Input: part model. Units: mm. Frame: model coordinates. A direction names the side the tool comes from. Give positions to 0.01 mm unless a question says otherwise; leave off trailing zeros. Order: outer loops, then holes, each group sorted by start corner. A loop starts at its lowest first (then second) coordinate and runs counter-clockwise, first axis right, second up. Notation, with made-up numbers: M 25,26 L 48,26 A16 ccw 48,43 Z; hole C 77,70 d7. An arc over 180 degrees is marked long. Use a Markdown table: item, result.
from build123d import *

# Parameters (mm, degrees)
SKETCH2_W           = 200
SKETCH2_H           = 205
BOSS_EXTRUDE1_DEPTH = 10
SKETCH3_W           = 10
SKETCH3_H           = 15
BOSS_EXTRUDE3_DEPTH = 160
SKETCH8_W           = 49.999986941
SKETCH8_H           = 10
BOSS_EXTRUDE4_DEPTH = 15
BOSS_EXTRUDE5_DEPTH = 15
SKETCH10_R          = 2
CUT_EXTRUDE1_DEPTH  = 10


with BuildPart() as part:
    # Sketch2 → Boss-Extrude1 (new body)
    with BuildSketch(Plane(origin=(0, 0, 0), x_dir=(1, 0, 0), z_dir=(0, 1, 0))):
        Rectangle(SKETCH2_W, SKETCH2_H)
    extrude(amount=BOSS_EXTRUDE1_DEPTH)

    # Sketch3 → Boss-Extrude3 (add)
    with BuildSketch(Plane(origin=(0, 0, 0), x_dir=(1, 0, 0), z_dir=(0, 1, 0))):
        Polygon((-14.947609587, -102.515331482), (-24.947604363, -102.525552471), (-24.962935845, -87.525560306), (-14.962941069, -87.515339317), align=None)
        with Locations((20.052382578, -95)):
            Rectangle(SKETCH3_W, SKETCH3_H)
    extrude(amount=BOSS_EXTRUDE3_DEPTH)

    # Sketch8 → Boss-Extrude4 (add)
    with BuildSketch(Plane.XY.offset(102.5)):
        with Locations((0.052389108, 145)):
            Rectangle(SKETCH8_W, SKETCH8_H)
    extrude(amount=BOSS_EXTRUDE4_DEPTH)

    # Sketch9 → Boss-Extrude5 (add)
    with BuildSketch(Plane.XY.offset(117.5)):
        Polygon((0.052389108, 150), (22.552389108, 150), (22.552389108, 140), (-22.447610892, 140), (-22.447610892, 150), align=None)
    extrude(amount=BOSS_EXTRUDE5_DEPTH)

    # Sketch10 → Cut-Extrude1 (cut)
    with BuildSketch(Plane(origin=(0, 150, 0), x_dir=(1, 0, 0), z_dir=(0, 1, 0))):
        with Locations(Location((17.552389108, -125, 0), (0, 0, 270))):
            Circle(SKETCH10_R)
        with Locations(Location((-17.447610892, -125, 0), (0, 0, 270))):
            Circle(SKETCH10_R)
    extrude(amount=-CUT_EXTRUDE1_DEPTH, mode=Mode.SUBTRACT)


solid = part.part
1) Mould query, pull axis X, two halves, no side actions, for faces 1 (the face through (1, 0, -1)), 2 (the face through (15.052, 84, 95)), 3 (the face through (25.052, 84, 96)), 4 (the face through (0, 145, 102.5)). Classes: released by +X, released by -X, zero draft, split by the parting line, or undercut.
Response values:
| item | result |
|---|---|
| face 1 | zero draft |
| face 2 | undercut |
| face 3 | released by +X |
| face 4 | undercut |
2) Cut plane B-B on y = 18. Return loops of the section in (x, z), and give its area (3 significant figures).
Response values:
| item | result |
|---|---|
| outline | M -24.96,87.53 L -14.96,87.52 L -14.95,102.52 L -24.95,102.53 Z; M 15.05,87.5 L 25.05,87.5 L 25.05,102.5 L 15.05,102.5 Z |
| area | 300 mm² |
3) Material intervals for line 1 (X direction, y = 142, z = 125); line 2 (Y direction, x = 65, z = 0); line 3 (Z direction, x = 24.5, y = 46.5), sorted ascending. Write a range as from..to.
Response values:
| item | result |
|---|---|
| line 1 | x = -22.45..-19.45, -15.45..15.55, 19.55..22.55 |
| line 2 | y = 0..10 |
| line 3 | z = 87.5..102.5 |
4) Cut plane C-C on z = -18. Return loops of the section in (x, y).
Response values:
| item | result |
|---|---|
| outline | M -100,0 L 100,0 L 100,10 L -100,10 Z |
5) First-contact query: pin 1 Ø5 at (x, y) = (19.5, 154) entering from +Z; pin 2 Ø5 at (x, z) = (-46, -27.5) entering from -Y; pin 3 Ø16.5 at (y, z) = (62, 94.5) entering from -X; pin 4 Ø3 at (y, z) = (147, 124.5) entering from -X. Flat tips, straight axial feed; report the tip coordinate or a pass-through.
Response values:
| item | result |
|---|---|
| pin 1 | stops at z = 102.5 |
| pin 2 | stops at y = 0 |
| pin 3 | stops at x = -24.96 |
| pin 4 | stops at x = -22.45 |
6) Cut plane D-D on x = 37.5. Return loops of the section in (y, z).
Response values:
| item | result |
|---|---|
| outline | M 0,-102.5 L 10,-102.5 L 10,102.5 L 0,102.5 Z |
7) Cut plane A-A on x = 1. Return loops of the section in (y, z).
Response values:
| item | result |
|---|---|
| outline | M 0,-102.5 L 10,-102.5 L 10,102.5 L 0,102.5 Z; M 140,102.5 L 150,102.5 L 150,132.5 L 140,132.5 Z |
8) Reachability of faces 5 (the face through (22.552, 145, 125)), 6 (the face through (0, 140, 117)), 7 (the face through (20, 84, 87.5)), 8 (the face through (20, 155, 102.5)) from +Z, -Z, +X, -X, +Y, -Y: full face, straight path, thin tool, end or side. Return the list, or none.
Response values:
| item | result |
|---|---|
| face 5 | +Z, +X, +Y, -Y |
| face 6 | +Z, +X, -X, -Y |
| face 7 | -Z, +X, -X, +Y |
| face 8 | +Z, +X, -X, +Y |
